Solid Edge part; units mm, degrees
sketch "Sketch1" plane through (0, 0, 0) normal (0, 0, 1) x (1, 0, 0)
  circle A0 centre (0, 0) radius 12.5
extrude "ExtrudedProtrusion_1" add sketch "Sketch1" along normal mid plane 10
sketch "Sketch2" plane through (0, 0, 0) normal (0, 0, 1) x (1, 0, 0)
  circle A0 centre (0, 0) radius 8
extrude "ExtrudedCutout_1" cut sketch "Sketch2" along normal mid plane 61.0802
sketch "Sketch3" plane through (0, 0, 0) normal (0, -1, 0) x (1, 0, 0)
  line L0 (14.5, 0) -> (14.5, 2)
  line L1 (14.5, 2) -> (-14.5, 1.0329)
  line L2 (-14.5, 1.0329) -> (-14.5, 0)
  line L3 (14.5, 0) -> (-14.5, 0)
  line L4 (0, 0) -> (14.5, 0)
revolve "RevolvedProtrusion_1" cut sketch "Sketch3" angle 360 about axis through (12.5, 0, 0) along (-1, 0, 0)
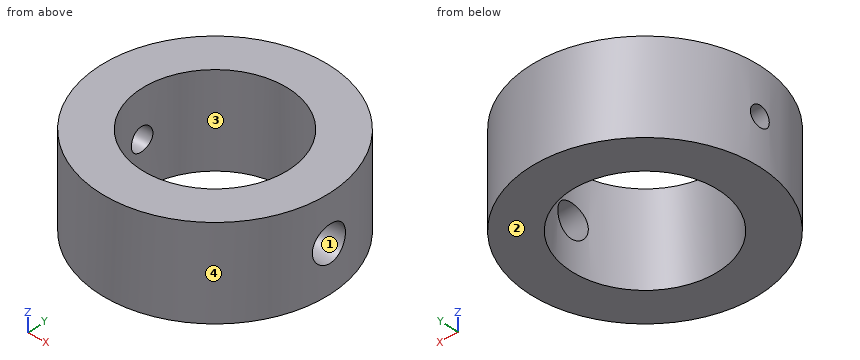
Geometry check sheet. Reference: the model listing, model coordinates, mm. Face numbers are marked on the shaded views. Give positions to 0.01 mm unless a question says otherwise; leave off trailing zeros. Order: outer loops, then holes, each group sorted by start corner. A loop starts at its lowest first (then second) coordinate and runs counter-clockwise, first axis right, second up.
1. Gauge pin test, flat ends, axial feed: pin 1 Ø5 at (x, z) = (7, -1.5) entering from +Y; pin 2 Ø3 at (x, z) = (3.5, 0) entering from -Y; pin 3 Ø2 at (x, z) = (-3.5, 0.5) entering from -Y; pin 4 Ø2 at (x, y) = (-2.5, -6) entering from -Z. Record the tip position at first contact, or that the pin passes through.
2. Thickness scan on L1, parallel to X at y = 0, z = 2.5; L2, parallel to X at y = 0, z = -1.75. Record the ranges inside material, lowest first.
3. Section check D-D, the plane y = 0. Enter the section's corners in (x, z).
4. Release check for a two-part mould opening along X. For the marked faces 1, 2, 3 and 4 record: pulls with the +X half, pulls with the -X half, needs draft (parallel to the pull), parting line crosses it, or undercut.
5. Section check A-A, the plane x = 0. Enter the section's corners in (y, z), and give its area (3 significant figures).
6. Section check C-C, the plane z = -4.25. Enter the section's corners in (x, y).
7. Section check B-B, the plane y = -7.5. Enter the section's corners in (x, z).
Values follow:
1. pin 1: stops at y = 11.66
1. pin 2: stops at y = -12.34
1. pin 3: stops at y = -12.25
1. pin 4: passes through
2. L1: x = -12.5 to -8, 8 to 12.5
2. L2: x = -12.5 to -8
3. outline: (-12.5, -5) - (-8, -5) - (-8, -1.25) - (-12.5, -1.1) - close; (-12.5, 1.1) - (-8, 1.25) - (-8, 5) - (-12.5, 5) - close; (8, -5) - (12.5, -5) - (12.5, -1.93) - (8, -1.78) - close; (8, 1.78) - (12.5, 1.93) - (12.5, 5) - (8, 5) - close
4. face 1: pulls with the +X half
4. face 2: needs draft
4. face 3: undercut
4. face 4: parting line crosses it
5. outline: (-12.5, -5) - (-8, -5) - (-8, 5) - (-12.5, 5) - close; (8, -5) - (12.5, -5) - (12.5, 5) - (8, 5) - close
5. area: 90.0 mm2
6. outline: circle Ø25 at (0, 0); hole circle Ø16 at (0, 0)
7. outline: (-10, -5) - (-2.78, -5) - (-2.78, 5) - (-10, 5) - close; (2.78, -5) - (10, -5) - (10, 5) - (2.78, 5) - close
